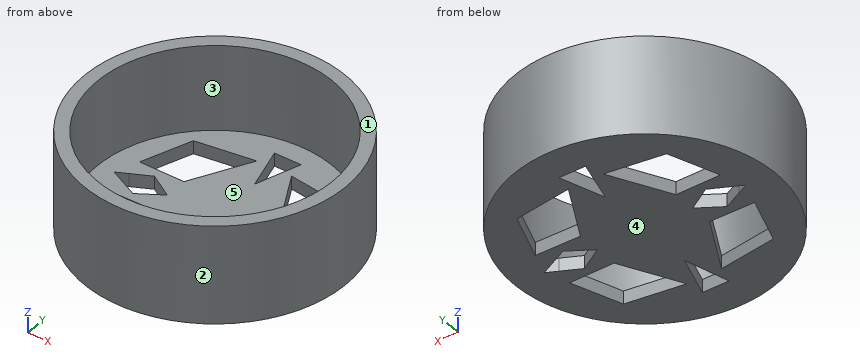
```python
from build123d import *

# Parameters (mm, degrees)
F0_R      = 20
F1_DEPTH  = 15
F2_R      = 18
F3_DEPTH  = 13
F9_DEPTH  = 8.7
F11_DEPTH = 11
F13_DEPTH = 22.4
F14_DEPTH = 4.9


# Not quite as in the source:
# - the program builds the solid bodies; features that only make, move or delete a surface that nothing else refers to are left out


with BuildPart() as f1:
    # F0 (on Top) → F1 (new body)
    with BuildSketch(Plane.XY):
        Circle(F0_R)
    extrude(amount=F1_DEPTH)

    # F2 (on face) → F3 (cut)
    with BuildSketch(Plane.XY.offset(15)):
        Circle(F2_R)
    extrude(amount=-F3_DEPTH, mode=Mode.SUBTRACT)

    # F8 (on face) → F9 (cut)
    with BuildSketch(Plane(origin=(0, 0, 0), x_dir=(1, 0, 0), z_dir=(0, 0, -1))):
        Polygon((-11.5306517109, 11.1294062808), (-14.2554212362, 3.5755613353), (-7.3548774235, 3.5121154506), (-2.6781838387, 12.3627316207), align=None)
        Polygon((7.3548774235, 3.5121154506), (14.2554212362, 3.5755613353), (11.5306517109, 11.1294062808), (2.6781838387, 12.3627316207), align=None)
        Polygon((11.5306517109, -11.1294062808), (14.2554212362, -3.5755613353), (7.3548774235, -3.5121154506), (2.6781838387, -12.3627316207), align=None)
        Polygon((-14.2554212362, -3.5755613353), (-11.5306517109, -11.1294062808), (-2.6781838387, -12.3627316207), (-7.3548774235, -3.5121154506), align=None)
    extrude(amount=-F9_DEPTH, mode=Mode.SUBTRACT)

    # F10 (on face) → F11 (cut)
    with BuildSketch(Plane(origin=(0, 0, 0), x_dir=(1, 0, 0), z_dir=(0, 0, -1))):
        Polygon((15.5360468029, 0), (13.8570014387, 0.8311709389), (10.9741548076, 2.2582546808), (7.3600309273, 0), (10.9741548076, -2.2582546808), (13.8570014387, -0.8311709389), align=None)
        Polygon((-10.9741548076, -2.2582546808), (-7.3600309273, 0), (-10.9741548076, 2.2582546808), (-13.8570014387, 0.8311709389), (-15.5360468029, 0), (-13.8570014387, -0.8311709389), align=None)
    extrude(amount=-F11_DEPTH, mode=Mode.SUBTRACT)

    # F12 (on face) → F13 (cut)
    with BuildSketch(Plane.XY.offset(2)):
        Polygon((2.2074584849, 14.9893220514), (-1.9000733737, 14.9893220514), (0, 8.2467701286), align=None)
        Polygon((-1.9000733737, -14.9893220514), (2.2074584849, -14.9893220514), (0, -8.2467701286), align=None)
    extrude(amount=F13_DEPTH, mode=Mode.SUBTRACT)

    # F12 (on face) → F14 (cut)
    with BuildSketch(Plane.XY.offset(2)):
        Polygon((2.2074584849, 14.9893220514), (-1.9000733737, 14.9893220514), (0, 8.2467701286), align=None)
        Polygon((-1.9000733737, -14.9893220514), (2.2074584849, -14.9893220514), (0, -8.2467701286), align=None)
    extrude(amount=-F14_DEPTH, mode=Mode.SUBTRACT)


solid = f1.part
```
Model file for the job. Use its own axes, mm. Face numbers are marked on the shaded views. A direction names the side the tool comes from. Coordinates: 2 decimals unless noted, no trailing zeros. Write each loop counter-clockwise with the first axis right and the second up, starting at its lowest first coordinate (ties: lowest second). Pieces come first, ordered by that corner, then holes. Notation, with made-up numbers: (59, -36) - (110, -36) arc R10 cw to (110, -20) - close; hole circle Ø6 at (73.5, 75.25). An arc over 180 degrees is marked (long way). One line per item, written item: value. Start each with the question number.
1. Probe line 1 (Y direction, x = 0, z = 9); line 2 (X direction, y = 8, z = 0.5); line 3 (X direction, y = 0.5, z = 6.5). List the from-to ranges inside material, lowest first. Write a range as from..to.
2. Flat gauge pins, fed straight in: pin 1 (2 mm diameter, centred on x = -10.5, y = -13, fed in from -Z); pin 2 (5 mm diameter, centred on x = 8.5, z = 13, fed in from -Y); pin 3 (1.6 mm diameter, centred on x = 1, z = 1, fed in from +Y); pin 4 (6 mm diameter, centred on x = -1.5, z = 4, fed in from -Y). Where does each tip first touch, or does it go through?
3. Tool access for the marked faces 4 and 5: list every direction of +Z, -Z, +X, -X, +Y, -Y with a clear straight run to the whole face (end or side of a thin tool).
4. Slice it at C-C (x = 3.5). Write the cut outline in (y, z).
5. Mould opens along Y. For the marked faces 1, 2 and 3 say: released by +Y, released by -Y, zero draft, split by the parting line, or undercut.
6. Slice it at D-D (z = 7.5). Write the cut outline in (x, y), plus the area to 3 significant figures.
7. Slice it at B-B (y = -14.5). Write the cut outline in (x, z).
8. Slice it at A-A (x = 9). Write the cut outline in (y, z), plus the area to 3 significant figures.
Answers below:
1. line 1: y = -20..-18, 18..20
1. line 2: x = -18.33..-12.66, -4.98..4.98, 12.66..18.33
1. line 3: x = -19.99..-17.99, 17.99..19.99
2. pin 1: stops at z = 0
2. pin 2: stops at y = -19.08
2. pin 3: stops at y = 20
2. pin 4: stops at y = -20
3. face 4: -Z, +X, -X, +Y, -Y
3. face 5: +Z
4. outline: (-19.69, 0) - (-12.25, 0) - (-12.25, 2) - (-17.66, 2) - (-17.66, 15) - (-19.69, 15) - close; (-10.81, 0) - (10.81, 0) - (10.81, 2) - (-10.81, 2) - close; (12.25, 0) - (19.69, 0) - (19.69, 15) - (17.66, 15) - (17.66, 2) - (12.25, 2) - close
5. face 1: zero draft
5. face 2: split by the parting line
5. face 3: undercut
6. outline: circle Ø40 at (0, 0); hole circle Ø36 at (0, 0)
6. area: 239 mm^2
7. outline: (-13.77, 0) - (-1.76, 0) - (-1.76, 2) - (-10.67, 2) - (-10.67, 15) - (-13.77, 15) - close; (2.05, 0) - (13.77, 0) - (13.77, 15) - (10.67, 15) - (10.67, 2) - (2.05, 2) - close
8. outline: (-17.86, 0) - (-11.48, 0) - (-11.48, 2) - (-15.59, 2) - (-15.59, 15) - (-17.86, 15) - close; (-3.53, 0) - (-1.02, 0) - (-1.02, 2) - (-3.53, 2) - close; (1.02, 0) - (3.53, 0) - (3.53, 2) - (1.02, 2) - close; (11.48, 0) - (17.86, 0) - (17.86, 15) - (15.59, 15) - (15.59, 2) - (11.48, 2) - close
8. area: 94.6 mm^2
